```python
from build123d import *

# Parameters (mm, degrees)
F1_DEPTH = 550


with BuildPart() as f1:
    # F0 (on Top) → F1 (new body)
    with BuildSketch(Plane.XY):
        with BuildLine():
            Line((-30, 50), (-50, 50))
            Line((-50, 50), (-50, 30))
            Line((-50, 30), (-44, 30))
            Line((-44, 30), (-44, 35))
            Line((-44, 35), (-37, 35))
            Line((-37, 35), (-37, 25.5))
            Line((-37, 25.5), (-30.97913, 25.5))
            ThreePointArc((-30.97913, 25.5), (-29.242641, 29.242641), (-25.5, 30.97913))
            ThreePointArc((-25.5, 30.97913), (-20.408156, 28.861991), (-19.195037, 23.482633))
            Line((-19.195037, 23.482633), (-12.5, 30.17767))
            Line((-12.5, 30.17767), (12.5, 30.17767))
            Line((12.5, 30.17767), (19.195037, 23.482633))
            ThreePointArc((19.195037, 23.482633), (29.242641, 29.242641), (23.482633, 19.195037))
            Line((23.482633, 19.195037), (30.17767, 12.5))
            Line((30.17767, 12.5), (30.17767, -12.5))
            Line((30.17767, -12.5), (23.482633, -19.195037))
            ThreePointArc((23.482633, -19.195037), (29.242641, -29.242641), (19.195037, -23.482633))
            Line((19.195037, -23.482633), (12.5, -30.17767))
            Line((12.5, -30.17767), (-12.5, -30.17767))
            Line((-12.5, -30.17767), (-19.195037, -23.482633))
            ThreePointArc((-19.195037, -23.482633), (-29.242641, -29.242641), (-23.482633, -19.195037))
            Line((-23.482633, -19.195037), (-30.17767, -12.5))
            Line((-30.17767, -12.5), (-30.17767, 12.5))
            Line((-30.17767, 12.5), (-23.482633, 19.195037))
            ThreePointArc((-23.482633, 19.195037), (-28.465904, 20.102295), (-30.97913, 24.5))
            Line((-30.97913, 24.5), (-37, 24.5))
            Line((-37, 24.5), (-37, 15))
            Line((-37, 15), (-44, 15))
            Line((-44, 15), (-44, 20))
            Line((-44, 20), (-50, 20))
            Line((-50, 20), (-50, -20))
            Line((-50, -20), (-44, -20))
            Line((-44, -20), (-44, -15))
            Line((-44, -15), (-37, -15))
            Line((-37, -15), (-37, -35))
            Line((-37, -35), (-44, -35))
            Line((-44, -35), (-44, -30))
            Line((-44, -30), (-50, -30))
            Line((-50, -30), (-50, -50))
            Line((-50, -50), (-30, -50))
            Line((-30, -50), (-30, -44))
            Line((-30, -44), (-35, -44))
            Line((-35, -44), (-35, -37))
            Line((-35, -37), (-15, -37))
            Line((-15, -37), (-15, -44))
            Line((-15, -44), (-20, -44))
            Line((-20, -44), (-20, -50))
            Line((-20, -50), (20, -50))
            Line((20, -50), (20, -44))
            Line((20, -44), (15, -44))
            Line((15, -44), (15, -37))
            Line((15, -37), (35, -37))
            Line((35, -37), (35, -44))
            Line((35, -44), (30, -44))
            Line((30, -44), (30, -50))
            Line((30, -50), (50, -50))
            Line((50, -50), (50, -30))
            Line((50, -30), (44, -30))
            Line((44, -30), (44, -35))
            Line((44, -35), (37, -35))
            Line((37, -35), (37, -15))
            Line((37, -15), (44, -15))
            Line((44, -15), (44, -20))
            Line((44, -20), (50, -20))
            Line((50, -20), (50, 20))
            Line((50, 20), (44, 20))
            Line((44, 20), (44, 15))
            Line((44, 15), (37, 15))
            Line((37, 15), (37, 35))
            Line((37, 35), (44, 35))
            Line((44, 35), (44, 30))
            Line((44, 30), (50, 30))
            Line((50, 30), (50, 50))
            Line((50, 50), (30, 50))
            Line((30, 50), (30, 44))
            Line((30, 44), (35, 44))
            Line((35, 44), (35, 37))
            Line((35, 37), (15, 37))
            Line((15, 37), (15, 44))
            Line((15, 44), (20, 44))
            Line((20, 44), (20, 50))
            Line((20, 50), (-20, 50))
            Line((-20, 50), (-20, 44))
            Line((-20, 44), (-15, 44))
            Line((-15, 44), (-15, 37))
            Line((-15, 37), (-25.5, 37))
            Line((-25.5, 37), (-35, 37))
            Line((-35, 37), (-35, 44))
            Line((-35, 44), (-30, 44))
            Line((-30, 44), (-30, 50))
        make_face()
    extrude(amount=F1_DEPTH)


solid = f1.part
```
Model file for the job. Use its own axes, mm. A direction names the side the tool comes from. Give positions to 0.01 mm unless a question says otherwise; leave off trailing zeros. Loops run counter-clockwise (first coordinate to the right, second up) from the corner with the lowest first, then second, coordinate; pieces in that order, holes last. Notation, with made-up numbers: (60.5, 10.5) -> (119.5, 10.5) arc R25 cw to (119.5, 27.5) -> close; hole circle Ø5 at (-29, -3). An arc over 180 degrees is marked (long way). Use CSV: the item, a comma, the result in double quotes. Start each with the question number.
1) Slice it at A-A on y = 5.5. Give the cut face in (x, z), plus the area to 3 significant figures.
2) Wall check: line 1 (Y direction, x = -39, z = 326.5); line 2 (X direction, y = -33, z = 121). Give the ranges that are in metal, low to high.
3) Mould opens along Y. For faces 3 (the flat face through (0, 50, 271)), 4 (the flat face through (-40, -50, 271)), 5 (the flat face through (-37, -25, 271)) say: released by +Y, released by -Y, zero draft, split by the parting line, or undercut.
4) Tool access for faces 1 (the flat face through (-34, 1, 550)), 2 (the flat face through (-37, 20, 271)): list every direction of +Z, -Z, +X, -X, +Y, -Y with a clear straight run to the whole face (end or side of a thin tool).
5) Flat gauge pin, fed straight in: pin 1 Ø1.5 at (y, z) = (24.5, 331.5) entering from -X. Where does the tip first touch, or does it go through?
Computed values:
1,outline,"(-50, 0) -> (-30.18, 0) -> (-30.18, 550) -> (-50, 550) -> close; (30.18, 0) -> (50, 0) -> (50, 550) -> (30.18, 550) -> close"
1,area,"21,800 mm^2"
2,line 1,"y = -50 to -35, -15 to 15, 35 to 50"
2,line 2,"x = -50 to -44, -37 to 37, 44 to 50"
3,face 3,"released by +Y"
3,face 4,"released by -Y"
3,face 5,"undercut"
4,face 1,"+Z, +X, -X, +Y, -Y"
4,face 2,"+Z, -Z"
5,pin 1,"stops at x = -37"
